```python
from build123d import *

# Parameters (mm, degrees)
SKETCH_1_W          = 166
SKETCH_1_H          = 138
EXTRUDE_1_DEPTH     = 3
SKETCH_2_W          = 166
SKETCH_2_H          = 138
SKETCH_2_W_2        = 159
SKETCH_2_H_2        = 131
EXTRUDE_2_DEPTH     = 40
CUT_EXTRUDE_4_REACH = 117.109
SKETCH_3_R          = 6.25
SKETCH_4_W          = 92
SKETCH_4_H          = 2.2
CUT_EXTRUDE_5_DEPTH = 1
SKETCH_5_W          = 92
SKETCH_5_H          = 2.2
CUT_EXTRUDE_6_DEPTH = 1


with BuildPart() as part:
    # 스케치1 → 보스-돌출1 (new body)
    with BuildSketch(Plane.XY):
        Rectangle(SKETCH_1_W, SKETCH_1_H)
    extrude(amount=EXTRUDE_1_DEPTH)

    # 스케치2 → 보스-돌출2 (add)
    with BuildSketch(Plane.XY.offset(3)):
        Rectangle(SKETCH_2_W, SKETCH_2_H)
        Rectangle(SKETCH_2_W_2, SKETCH_2_H_2, mode=Mode.SUBTRACT)
    extrude(amount=EXTRUDE_2_DEPTH)

    # 스케치3 → 컷-돌출4 (cut, up to next)
    with BuildSketch(Plane.XY.offset(3), mode=Mode.PRIVATE) as cut_extrude_4_sk1:
        with Locations((-58, 44)):
            Circle(SKETCH_3_R)
    cut_extrude_4_tool1 = extrude(cut_extrude_4_sk1.sketch, amount=-CUT_EXTRUDE_4_REACH, mode=Mode.PRIVATE) & part.part
    # 스케치3 → 컷-돌출4 (cut, up to next)
    with BuildSketch(Plane.XY.offset(3), mode=Mode.PRIVATE) as cut_extrude_4_sk2:
        with Locations((-58, -44)):
            Circle(SKETCH_3_R)
    cut_extrude_4_tool2 = extrude(cut_extrude_4_sk2.sketch, amount=-CUT_EXTRUDE_4_REACH, mode=Mode.PRIVATE) & part.part
    # 스케치3 → 컷-돌출4 (cut, up to next)
    with BuildSketch(Plane.XY.offset(3), mode=Mode.PRIVATE) as cut_extrude_4_sk3:
        with Locations((58, -44)):
            Circle(SKETCH_3_R)
    cut_extrude_4_tool3 = extrude(cut_extrude_4_sk3.sketch, amount=-CUT_EXTRUDE_4_REACH, mode=Mode.PRIVATE) & part.part
    # 스케치3 → 컷-돌출4 (cut, up to next)
    with BuildSketch(Plane.XY.offset(3), mode=Mode.PRIVATE) as cut_extrude_4_sk4:
        with Locations((58, 44)):
            Circle(SKETCH_3_R)
    cut_extrude_4_tool4 = extrude(cut_extrude_4_sk4.sketch, amount=-CUT_EXTRUDE_4_REACH, mode=Mode.PRIVATE) & part.part
    add(cut_extrude_4_tool1.solids().sort_by_distance((-58, 44, 3))[0], mode=Mode.SUBTRACT)
    add(cut_extrude_4_tool2.solids().sort_by_distance((-58, -44, 3))[0], mode=Mode.SUBTRACT)
    add(cut_extrude_4_tool3.solids().sort_by_distance((58, -44, 3))[0], mode=Mode.SUBTRACT)
    add(cut_extrude_4_tool4.solids().sort_by_distance((58, 44, 3))[0], mode=Mode.SUBTRACT)

    # 스케치4 → 컷-돌출5 (cut)
    with BuildSketch(Plane.XZ.offset(-65.5)):
        with Locations((0, 40)):
            Rectangle(SKETCH_4_W, SKETCH_4_H)
    extrude(amount=-CUT_EXTRUDE_5_DEPTH, mode=Mode.SUBTRACT)

    # 스케치5 → 컷-돌출6 (cut)
    with BuildSketch(Plane(origin=(0, -65.5, 0), x_dir=(1, 0, 0), z_dir=(0, 1, 0))):
        with Locations((-0.014955436, -40)):
            Rectangle(SKETCH_5_W, SKETCH_5_H)
    extrude(amount=-CUT_EXTRUDE_6_DEPTH, mode=Mode.SUBTRACT)


solid = part.part
```
Geometry: final body of the model. Coordinates: model frame, mm. A direction names the side the tool comes from. Coordinates: 2 decimals unless noted, no trailing zeros. Write each loop counter-clockwise with the first axis right and the second up, starting at its lowest first coordinate (ties: lowest second). Pieces come first, ordered by that corner, then holes. Notation, with made-up numbers: M -2.5,10.25 L 35.5,10.25 A34 ccw 35.5,46.25 Z; hole C -29.75,21.25 d5. An arc over 180 degrees is marked long. Answer as CSV lines item,"result". Start each with the question number.
Q1. Mould query, pull axis Y, two halves, no side actions, for faces 1 (the flat face through (-1, 69, 21)), 2 (the flat face through (-1, -69, 21)), 3 (the cylindrical face through (63.96, 45.88, 1.52)). Classes: released by +Y, released by -Y, zero draft, split by the parting line, or undercut.
Q2. Cut plane A-A on y = 44. Return the cut outline in (x, z).
Q3. Reachability of faces 4 (the cylindrical face through (-52.04, -42.12, 1.52)), 5 (the flat face through (-79.5, -1, 23)) from +Z, -Z, +X, -X, +Y, -Y: full face, straight path, thin tool, end or side. Return the list, or none.
Q4. Line query: line 1 (Y direction, x = -58, z = 1); line 2 (X direction, y = -54, z = 14.5); line 3 (Y direction, x = -22, z = 22). Output: solid intervals per line, ascending. Write a range as from..to.
Q5. Cut plane C-C on x = -27.5. Return the cut outline in (y, z), then the cut area to 3 significant figures.
Q6. Cut plane B-B on z = 19.5. Return the cut outline in (x, y), then the cut area to 3 significant figures.
Q7. Cut plane D-D on x = 58. Return the cut outline in (y, z), then the cut area to 3 significant figures.
Q8. Pin query (flat end, axial travel): P1, Ø20, axis at x = -58, y = 44, coming from the +Z side; P2, Ø16, axis at x = 58, y = 44, coming from the -Z side. Return the tip coordinate at first contact, or that it passes through.
Findings below:
1,face 1,"released by +Y"
1,face 2,"released by -Y"
1,face 3,"undercut"
2,outline,"M -83,0 L -64.25,0 L -64.25,3 L -79.5,3 L -79.5,43 L -83,43 Z; M -51.75,0 L 51.75,0 L 51.75,3 L -51.75,3 Z; M 64.25,0 L 83,0 L 83,43 L 79.5,43 L 79.5,3 L 64.25,3 Z"
3,face 4,"+Z, -Z"
3,face 5,"+Z"
4,line 1,"y = -69..-50.25, -37.75..37.75, 50.25..69"
4,line 2,"x = -83..-79.5, 79.5..83"
4,line 3,"y = -69..-65.5, 65.5..69"
5,outline,"M -69,0 L 69,0 L 69,43 L 65.5,43 L 65.5,41.1 L 66.5,41.1 L 66.5,38.9 L 65.5,38.9 L 65.5,3 L -65.5,3 L -65.5,38.9 L -66.5,38.9 L -66.5,41.1 L -65.5,41.1 L -65.5,43 L -69,43 Z"
5,area,"690 mm2"
6,outline,"M -83,-69 L 83,-69 L 83,69 L -83,69 Z; hole M -79.5,-65.5 L 79.5,-65.5 L 79.5,65.5 L -79.5,65.5 Z"
6,area,"2,080 mm2"
7,outline,"M -69,0 L -50.25,0 L -50.25,3 L -65.5,3 L -65.5,43 L -69,43 Z; M -37.75,0 L 37.75,0 L 37.75,3 L -37.75,3 Z; M 50.25,0 L 69,0 L 69,43 L 65.5,43 L 65.5,3 L 50.25,3 Z"
7,area,"619 mm2"
8,P1,"stops at z = 3"
8,P2,"stops at z = 0"
